Work out the finished part from the listing and answer in its coordinate system (mm). A direction names the side the tool comes from. Round coordinates to 2 decimals unless told otherwise and drop trailing zeros. Order: outer loops, then holes, each group sorted by start corner. A loop starts at its lowest first (then second) coordinate and runs counter-clockwise, first axis right, second up. Notation, with made-up numbers: M -11,67 L 39,67 A20 cw 39,100 Z; hole C 25,-0.5 d11. An arc over 180 degrees is marked long. Return JSON: item names as keys, results as strings.
from build123d import *
from OCP.BRepFilletAPI import BRepFilletAPI_MakeChamfer

# Parameters (mm, degrees)
SKETCH1_R                = 29.468618182
SKETCH1_R_2              = 6.35
BOSS_EXTRUDE1_DEPTH      = 3.175
CHAMFER1_SIZE            = 2.54
CHAMFER1_SIZE2           = 0.680590949
CUT_EXTRUDE2_DEPTH       = 42.795688056
BOSS_EXTRUDE2_DEPTH      = 7.112
BOSS_EXTRUDE2_DEPTH_BACK = 10.287
SKETCH4_R                = 21.59
SKETCH4_R_2              = 6.35


with BuildPart() as part:
    # Sketch1 → Boss-Extrude1 (new body)
    with BuildSketch(Plane(origin=(0, 0, 0), x_dir=(1, 0, 0), z_dir=(0, 1, 0))):
        with Locations(Location((0, 0, 0), (0, 0, 270))):
            Circle(SKETCH1_R)
        with Locations(Location((0, 0, 0), (0, 0, 270))):
            Circle(SKETCH1_R_2, mode=Mode.SUBTRACT)
    extrude(amount=BOSS_EXTRUDE1_DEPTH)

    # Chamfer1: one chamfer whose edges measure the first distance from different faces: ONE call of the kernel's chamfer builder (chamfer() names one face for all edges)
    chamfer1_edges_1 = [part.edges().sort_by_distance(p)[0] for p in [
        (0, 0, -29.468618182),
    ]]
    chamfer1_side_1 = [part.faces().sort_by_distance(p)[0] for p in [
        (0, 0, -28.635119792),
    ]]
    chamfer1_edges_2 = [part.edges().sort_by_distance(p)[0] for p in [
        (0, 3.175, -29.468618182),
    ]]
    chamfer1_side_2 = [part.faces().sort_by_distance(p)[0] for p in [
        (0, 3.175, -28.635119792),
    ]]
    chamfer1 = BRepFilletAPI_MakeChamfer(part.part.solid().wrapped)
    for e in chamfer1_edges_1:
        chamfer1.Add(CHAMFER1_SIZE, CHAMFER1_SIZE2, e.wrapped, chamfer1_side_1[0].wrapped)  # the first distance lies on this face
    for e in chamfer1_edges_2:
        chamfer1.Add(CHAMFER1_SIZE, CHAMFER1_SIZE2, e.wrapped, chamfer1_side_2[0].wrapped)  # the first distance lies on this face
    add(Compound.cast(chamfer1.Shape()), mode=Mode.REPLACE)

    # Sketch3 → Cut-Extrude2 (cut, through all)
    with BuildSketch(Plane(origin=(0, 3.175, 0), x_dir=(1, 0, 0), z_dir=(0, 1, 0))):
        with BuildLine():
            Line((2.362951064, 26.551174329), (3.355071849, 29.277003782))
            ThreePointArc((3.355071849, 29.277003782), (0, 29.468618182), (-3.355071849, 29.277003782))
            Line((-3.355071849, 29.277003782), (-2.362951064, 26.551174329))
            ThreePointArc((-2.362951064, 26.551174329), (0, 24.896618182), (2.362951064, 26.551174329))
        make_face()
        with BuildLine():
            Line((6.860588771, 25.758119452), (6.860588771, 28.658886567))
            ThreePointArc((6.860588771, 28.658886567), (10.078861014, 27.69144305), (13.166061288, 26.363882258))
            Line((13.166061288, 26.363882258), (11.301484128, 24.141765729))
            ThreePointArc((11.301484128, 24.141765729), (8.515144919, 23.395168388), (6.860588771, 25.758119452))
        make_face()
        with BuildLine():
            Line((15.256640349, 21.85825522), (16.248761134, 24.584084672))
            ThreePointArc((16.248761134, 24.584084672), (18.942062642, 22.574271205), (21.389029426, 20.270887444))
            Line((21.389029426, 20.270887444), (18.876891414, 18.820503887))
            ThreePointArc((18.876891414, 18.820503887), (16.00323769, 19.071916011), (15.256640349, 21.85825522))
        make_face()
        with BuildLine():
            Line((21.812515937, 15.321962814), (23.677093097, 17.544079343))
            ThreePointArc((23.677093097, 17.544079343), (25.52057196, 14.734309091), (27.032164946, 11.732924438))
            Line((27.032164946, 11.732924438), (24.175467002, 11.229211515))
            ThreePointArc((24.175467002, 11.229211515), (21.561103814, 12.448309091), (21.812515937, 15.321962814))
        make_face()
        with BuildLine():
            Line((25.737480185, 6.937615565), (28.249618197, 8.387999123))
            ThreePointArc((28.249618197, 8.387999123), (29.020923656, 5.117171846), (29.414822422, 1.779797586))
            Line((29.414822422, 1.779797586), (26.558124477, 2.283510509))
            ThreePointArc((26.558124477, 2.283510509), (24.518382609, 4.323252377), (25.737480185, 6.937615565))
        make_face()
        with BuildLine():
            Line((26.558124477, -2.283510509), (29.414822422, -1.779797586))
            ThreePointArc((29.414822422, -1.779797586), (29.020923656, -5.117171846), (28.249618197, -8.387999123))
            Line((28.249618197, -8.387999123), (25.737480185, -6.937615565))
            ThreePointArc((25.737480185, -6.937615565), (24.518382609, -4.323252377), (26.558124477, -2.283510509))
        make_face()
        with BuildLine():
            Line((24.175467002, -11.229211515), (27.032164946, -11.732924438))
            ThreePointArc((27.032164946, -11.732924438), (25.52057196, -14.734309091), (23.677093097, -17.544079343))
            Line((23.677093097, -17.544079343), (21.812515937, -15.321962814))
            ThreePointArc((21.812515937, -15.321962814), (21.561103814, -12.448309091), (24.175467002, -11.229211515))
        make_face()
        with BuildLine():
            Line((18.876891414, -18.820503887), (21.389029426, -20.270887444))
            ThreePointArc((21.389029426, -20.270887444), (18.942062642, -22.574271205), (16.248761134, -24.584084672))
            Line((16.248761134, -24.584084672), (15.256640349, -21.85825522))
            ThreePointArc((15.256640349, -21.85825522), (16.00323769, -19.071916011), (18.876891414, -18.820503887))
        make_face()
        with BuildLine():
            Line((11.301484128, -24.141765729), (13.166061288, -26.363882258))
            ThreePointArc((13.166061288, -26.363882258), (10.078861014, -27.69144305), (6.860588771, -28.658886567))
            Line((6.860588771, -28.658886567), (6.860588771, -25.758119452))
            ThreePointArc((6.860588771, -25.758119452), (8.515144919, -23.395168388), (11.301484128, -24.141765729))
        make_face()
        with BuildLine():
            Line((2.362951064, -26.551174329), (3.355071849, -29.277003782))
            ThreePointArc((3.355071849, -29.277003782), (0, -29.468618182), (-3.355071849, -29.277003782))
            Line((-3.355071849, -29.277003782), (-2.362951064, -26.551174329))
            ThreePointArc((-2.362951064, -26.551174329), (0, -24.896618182), (2.362951064, -26.551174329))
        make_face()
        with BuildLine():
            Line((-6.860588771, -25.758119452), (-6.860588771, -28.658886567))
            ThreePointArc((-6.860588771, -28.658886567), (-10.078861014, -27.69144305), (-13.166061288, -26.363882258))
            Line((-13.166061288, -26.363882258), (-11.301484128, -24.141765729))
            ThreePointArc((-11.301484128, -24.141765729), (-8.515144919, -23.395168388), (-6.860588771, -25.758119452))
        make_face()
        with BuildLine():
            Line((-15.256640349, -21.85825522), (-16.248761134, -24.584084672))
            ThreePointArc((-16.248761134, -24.584084672), (-18.942062642, -22.574271205), (-21.389029426, -20.270887444))
            Line((-21.389029426, -20.270887444), (-18.876891414, -18.820503887))
            ThreePointArc((-18.876891414, -18.820503887), (-16.00323769, -19.071916011), (-15.256640349, -21.85825522))
        make_face()
        with BuildLine():
            Line((-21.812515937, -15.321962814), (-23.677093097, -17.544079343))
            ThreePointArc((-23.677093097, -17.544079343), (-25.52057196, -14.734309091), (-27.032164946, -11.732924438))
            Line((-27.032164946, -11.732924438), (-24.175467002, -11.229211515))
            ThreePointArc((-24.175467002, -11.229211515), (-21.561103814, -12.448309091), (-21.812515937, -15.321962814))
        make_face()
        with BuildLine():
            Line((-25.737480185, -6.937615565), (-28.249618197, -8.387999123))
            ThreePointArc((-28.249618197, -8.387999123), (-29.020923656, -5.117171846), (-29.414822422, -1.779797586))
            Line((-29.414822422, -1.779797586), (-26.558124477, -2.283510509))
            ThreePointArc((-26.558124477, -2.283510509), (-24.518382609, -4.323252377), (-25.737480185, -6.937615565))
        make_face()
        with BuildLine():
            Line((-26.558124477, 2.283510509), (-29.414822422, 1.779797586))
            ThreePointArc((-29.414822422, 1.779797586), (-29.020923656, 5.117171846), (-28.249618197, 8.387999123))
            Line((-28.249618197, 8.387999123), (-25.737480185, 6.937615565))
            ThreePointArc((-25.737480185, 6.937615565), (-24.518382609, 4.323252377), (-26.558124477, 2.283510509))
        make_face()
        with BuildLine():
            Line((-24.175467002, 11.229211515), (-27.032164946, 11.732924438))
            ThreePointArc((-27.032164946, 11.732924438), (-25.52057196, 14.734309091), (-23.677093097, 17.544079343))
            Line((-23.677093097, 17.544079343), (-21.812515937, 15.321962814))
            ThreePointArc((-21.812515937, 15.321962814), (-21.561103814, 12.448309091), (-24.175467002, 11.229211515))
        make_face()
        with BuildLine():
            Line((-18.876891414, 18.820503887), (-21.389029426, 20.270887444))
            ThreePointArc((-21.389029426, 20.270887444), (-18.942062642, 22.574271205), (-16.248761134, 24.584084672))
            Line((-16.248761134, 24.584084672), (-15.256640349, 21.85825522))
            ThreePointArc((-15.256640349, 21.85825522), (-16.00323769, 19.071916011), (-18.876891414, 18.820503887))
        make_face()
        with BuildLine():
            Line((-11.301484128, 24.141765729), (-13.166061288, 26.363882258))
            ThreePointArc((-13.166061288, 26.363882258), (-10.078861014, 27.69144305), (-6.860588771, 28.658886567))
            Line((-6.860588771, 28.658886567), (-6.860588771, 25.758119452))
            ThreePointArc((-6.860588771, 25.758119452), (-8.515144919, 23.395168388), (-11.301484128, 24.141765729))
        make_face()
    extrude(amount=-CUT_EXTRUDE2_DEPTH, mode=Mode.SUBTRACT)

    # Sketch4 → Boss-Extrude2 (add, two sides: drawn at the far end of the back side and taken through both)
    with BuildSketch(Plane(origin=(0, 3.175, 0), x_dir=(1, 0, 0), z_dir=(0, 1, 0)).offset(-BOSS_EXTRUDE2_DEPTH_BACK)):
        with Locations(Location((0, 0, 0), (0, 0, 270))):
            Circle(SKETCH4_R)
        with Locations(Location((0, 0, 0), (0, 0, 270))):
            Circle(SKETCH4_R_2, mode=Mode.SUBTRACT)
    extrude(amount=BOSS_EXTRUDE2_DEPTH + BOSS_EXTRUDE2_DEPTH_BACK)


solid = part.part
Item 1: Which of the six approach directions +Z, -Z, +X, -X, +Y, -Y give full straight-line access (tool end or side, diameter ignored) to faces 4 (the flat face through (12.25, 1.61, -25.27)), 5 (the flat face through (22.76, 1.61, 16.45)), 6 (the flat face through (-15.746, 1.61, 23.202))?
Output:
{"face 4": "-Z, +Y, -Y", "face 5": "+X, +Y, -Y", "face 6": "-X, +Y, -Y"}
Item 2: Consider line 1 along X through (y, z) = (-1, 0); line 2 along X through (y, z) = (1.5, -24); line 3 along Z through (x, y) = (-10.5, 3.5). Determine where each line is inside the solid, lowest interval first. Write a range as [from, to].
Output:
{"line 1": "x = [-21.59, -6.35], [6.35, 21.59]", "line 2": "x = [-16.04, -11.17], [-7.58, 7.58], [11.17, 16.04]", "line 3": "z = [-18.86, 18.86]"}
Item 3: The mould has two halves that part along X. Classify faces 1 (the flat face through (12.221, 1.61, 25.237)), 2 (the conical face through (14.08, 0.345, 24.453)), 3 (the conical face through (-14.137, 0.345, 24.42)): pulls with the +X half, pulls with the -X half, needs draft (parallel to the pull), parting line crosses it, or undercut.
Output:
{"face 1": "undercut", "face 2": "pulls with the +X half", "face 3": "pulls with the -X half"}
Item 4: Find section A-A (x = 0). Determine the outline of the cut face in (y, z) (3 decimals), plus the area to 3 significant figures.
Output:
{"outline": "M -7.112,-21.59 L 0,-21.59 L 0,-24.897 L 3.175,-24.897 L 3.175,-21.59 L 10.287,-21.59 L 10.287,-6.35 L -7.112,-6.35 Z; M -7.112,6.35 L 10.287,6.35 L 10.287,21.59 L 3.175,21.59 L 3.175,24.897 L 0,24.897 L 0,21.59 L -7.112,21.59 Z", "area": "551 mm^2"}
Item 5: Find section C-C (y = 6.25). Determine the outline of the cut face in (x, z).
Output:
{"outline": "C 0,0 d43.18; hole C 0,0 d12.7"}
Item 6: Each of these flat-tipped pins is pushed along its axis until it touches: pin 1 (3 mm diameter, centred on y = -1, z = -4, fed in from -X); pin 2 (4 mm diameter, centred on x = -11.5, y = 4, fed in from +Z); pin 3 (3 mm diameter, centred on y = 3, z = 11.5, fed in from +X); pin 4 (8 mm diameter, centred on x = 3, z = -3.5, fed in from -Y). Where does it stop, or does it pass through?
Output:
{"pin 1": "stops at x = -25.32", "pin 2": "stops at z = 26.07", "pin 3": "stops at x = 27.69", "pin 4": "stops at y = -7.11"}
Item 7: Find section B-B (z = 0). Determine the outline of the cut face in (x, y) (3 decimals), plus the area to 3 significant figures.
Output:
{"outline": "M -29.469,0.681 L -26.929,0 L -21.59,0 L -21.59,-7.112 L -6.35,-7.112 L -6.35,10.287 L -21.59,10.287 L -21.59,3.175 L -26.929,3.175 L -29.469,2.494 Z; M 6.35,-7.112 L 21.59,-7.112 L 21.59,0 L 26.929,0 L 29.469,0.681 L 29.469,2.494 L 26.929,3.175 L 21.59,3.175 L 21.59,10.287 L 6.35,10.287 Z", "area": "577 mm^2"}
